Check sheet for the modelled part. Datum: model origin and axes. Units: mm. Round coordinates to 2 decimals unless told otherwise and drop trailing zeros. Order: outer loops, then holes, each group sorted by start corner. A loop starts at its lowest first (then second) coordinate and runs counter-clockwise, first axis right, second up.
Q1. Cross-section at C-C on y = 0.5. Record the cut outline in (x, z).
Q2. Scan lines: probe 1 along Y at (x, z) = (-52, 3.75); probe 2 along Y at (x, z) = (-91, 8); probe 3 along Y at (x, z) = (-83, 8). Record each from-to range of solid material in increasing order.
Q3. Cross-section at A-A on z = 6.75. Record the cut outline in (x, y), then the cut area to 3 significant figures.
Q4. Depth check by flat-ended pin: P1, Ø1, axis at x = -46, y = 2.5, coming from the -Z side; P2, Ø2.5, axis at x = -90, y = 16, coming from the +Z side. Enter the tip coordinate at first touch or a pass-through.
Q5. Cross-section at B-B on x = 54. Record the cut outline in (y, z), then the cut area to 3 significant figures.
from build123d import *

# Parameters (mm, degrees)
BOSS_EXTRUDE1_DEPTH = 10
SKETCH2_R           = 1.55
CUT_EXTRUDE1_DEPTH  = 115.455231423
CUT_EXTRUDE2_REACH  = 116.455
SKETCH3_R           = 1.55


with BuildPart() as part:
    # Sketch1 → Boss-Extrude1 (new body)
    with BuildSketch(Plane.XY):
        Polygon((110, -30), (110, -10), (-30, 30), (-110, 30), (-110, -30), align=None)
    extrude(amount=BOSS_EXTRUDE1_DEPTH)

    # Sketch2 → Cut-Extrude1 (cut, through all)
    with BuildSketch(Plane.XY.offset(10)):
        with Locations((-90, 16)):
            Circle(SKETCH2_R)
        with Locations((-52, 16)):
            Circle(SKETCH2_R)
        with Locations((-90, -3)):
            Circle(SKETCH2_R)
        with Locations((-52, -3)):
            Circle(SKETCH2_R)
    extrude(amount=-CUT_EXTRUDE1_DEPTH, mode=Mode.SUBTRACT)

    # Sketch3 → Cut-Extrude2 (cut, up to next)
    with BuildSketch(Plane.XY.offset(10), mode=Mode.PRIVATE) as cut_extrude2_sk1:
        with Locations((-83, 26)):
            Circle(SKETCH3_R)
    cut_extrude2_tool1 = extrude(cut_extrude2_sk1.sketch, amount=-CUT_EXTRUDE2_REACH, mode=Mode.PRIVATE) & part.part
    add(cut_extrude2_tool1.solids().sort_by_distance((-83, 26, 10))[0], mode=Mode.SUBTRACT)


solid = part.part
Results found:
1. outline: (-110, 0) - (73.25, 0) - (73.25, 10) - (-110, 10) - close
2. probe 1: y = -30 to -4.55, -1.45 to 14.45, 17.55 to 30
2. probe 2: y = -30 to -4.18, -1.82 to 14.82, 17.18 to 30
2. probe 3: y = -30 to 24.45, 27.55 to 30
3. outline: (-110, -30) - (110, -30) - (110, -10) - (-30, 30) - (-110, 30) - close; hole circle Ø3.1 at (-90, -3); hole circle Ø3.1 at (-90, 16); hole circle Ø3.1 at (-83, 26); hole circle Ø3.1 at (-52, -3); hole circle Ø3.1 at (-52, 16)
3. area: 10,400 mm2
4. P1: stops at z = 0
4. P2: passes through
5. outline: (-30, 0) - (6, 0) - (6, 10) - (-30, 10) - close
5. area: 360 mm2
